Check sheet for the modelled part. Datum: model origin and axes. Units: mm. Coordinates: 2 decimals unless noted, no trailing zeros. Loops run counter-clockwise (first coordinate to the right, second up) from the corner with the lowest first, then second, coordinate; pieces in that order, holes last. Notation, with made-up numbers: M 89.5,28.5 L 93.5,28.5 A21 cw 93.5,58.5 Z; hole C -18.75,-18 d3. An arc over 180 degrees is marked long. Write each question's results on one line, items separated by ' | '. Start each with the question number.
from build123d import *

# Parameters (mm, degrees)
F0_W          = 1500
F0_H          = 100
F1_DEPTH      = 50
F2_T          = -3.25
F3_DEPTH      = 25
F3_DEPTH_BACK = 25


with BuildPart() as f1:
    # F0 (on Front) → F1 (new body)
    with BuildSketch(Plane.XZ):
        with Locations((9.0955580262, -3.9434796199)):
            Rectangle(F0_W, F0_H)
    extrude(amount=F1_DEPTH)

    # F2
    f2_openings = [f1.faces().sort_by_distance(p)[0] for p in [
        (759.095558, -25, -3.94348),
    ]]
    offset(amount=F2_T, openings=f2_openings)

    # F3 (cut, two sides): a face of the model
    f3_faces = [f1.faces().sort_by_distance(p)[0] for p in [
        (-737.6544419738, -25, -3.9434796199),
    ]]
    extrude(f3_faces, amount=-F3_DEPTH, mode=Mode.SUBTRACT)
    extrude(f3_faces, amount=F3_DEPTH_BACK, mode=Mode.SUBTRACT)


solid = f1.part
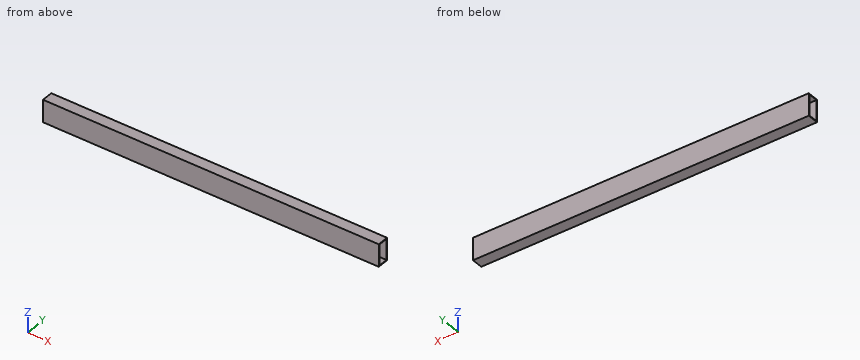
1) Thickness scan on probe 1 along Z at (x, y) = (289.5, -4); probe 2 along Y at (x, z) = (320, 5). Record the ranges inside material, lowest first.
2) Gauge pin test, flat ends, axial feed: P1, Ø6, axis at y = -42.5, z = 20, coming from the -X side; P2, Ø8, axis at x = 540, z = 32, coming from the +Y side. Record the tip position at first contact, or that the pin passes through.
3) Section check A-A (z = -35.5). Enter the section's corners in (x, y), then the cut area to 3 significant figures.
4) Section check C-C (x = 665). Enter the section's corners in (y, z).
5) Section check B-B (y = -18). Enter the section's corners in (x, z).
Return value:
1) probe 1: z = -53.94 to -50.69, 42.81 to 46.06 | probe 2: y = -50 to -46.75, -3.25 to 0
2) P1: passes through | P2: stops at y = 0
3) outline: M -740.9,-50 L 759.1,-50 L 759.1,-46.75 L -740.9,-46.75 Z; M -740.9,-3.25 L 759.1,-3.25 L 759.1,0 L -740.9,0 Z | area: 9,750 mm2
4) outline: M -50,-53.94 L 0,-53.94 L 0,46.06 L -50,46.06 Z; hole M -46.75,-50.69 L -3.25,-50.69 L -3.25,42.81 L -46.75,42.81 Z
5) outline: M -740.9,-53.94 L 759.1,-53.94 L 759.1,-50.69 L -740.9,-50.69 Z; M -740.9,42.81 L 759.1,42.81 L 759.1,46.06 L -740.9,46.06 Z
